Read the model definition and answer for the solid it produces. Units are mm, in the model's axes. A direction names the side the tool comes from. Coordinates: 2 decimals unless noted, no trailing zeros. Write each loop counter-clockwise with the first axis right and the second up, starting at its lowest first coordinate (ties: lowest second). Pieces come first, ordered by that corner, then holes. Notation, with made-up numbers: (-4, 14) - (41, 14) arc R13 ccw to (41, 29) - close; hole circle Ø7 at (-26.75, 47.25). An arc over 180 degrees is marked (long way). Use a Markdown table: item, result.
from build123d import *

# Parameters (mm, degrees)
SKETCH2_W            = 54.6
SKETCH2_H            = 28
SKETCH2_R            = 2.04
SKETCH2_W_2          = 40.6
SKETCH2_H_2          = 20.5
BOSS_EXTRUDE1_DEPTH  = 7.5
SKETCH3_W            = 40.6
SKETCH3_H            = 3.75
BOSS_EXTRUDE2_DEPTH  = 18.4
SKETCH7_W            = 74.600133011
SKETCH7_H            = 74.600133011
BOSS_EXTRUDE4_DEPTH  = 5
CUT_EXTRUDE2_DEPTH   = 5
SKETCH9_R            = 1.55
CUT_EXTRUDE3_DEPTH   = 16
FILLET3_R            = 1
FILLET3_OF_MIRROR4_R = 1
FILLET4_R            = 3


# Read off the part's stored shape, not the designer's step: Mirror5
with BuildPart() as part:
    # Sketch2 → Boss-Extrude1 (new body)
    with BuildSketch(Plane.XY):
        Rectangle(SKETCH2_W, SKETCH2_H)
        with Locations((23.85, 4.9)):
            Circle(SKETCH2_R, mode=Mode.SUBTRACT)
        with Locations(Location((23.85, -4.9, 0), (0, 0, 180))):
            Circle(SKETCH2_R, mode=Mode.SUBTRACT)
        with Locations((-23.85, -4.9)):
            Circle(SKETCH2_R, mode=Mode.SUBTRACT)
        with Locations(Location((-23.85, 4.9, 0), (0, 0, 180))):
            Circle(SKETCH2_R, mode=Mode.SUBTRACT)
        Rectangle(SKETCH2_W_2, SKETCH2_H_2, mode=Mode.SUBTRACT)
    extrude(amount=BOSS_EXTRUDE1_DEPTH)

    # Sketch3 → Boss-Extrude2 (add)
    with BuildSketch(Plane.XY.offset(7.5)):
        with Locations((0, 12.125)):
            Rectangle(SKETCH3_W, SKETCH3_H)
        with Locations((0, -12.125)):
            Rectangle(SKETCH3_W, SKETCH3_H)
    extrude(amount=BOSS_EXTRUDE2_DEPTH)

    # Sketch7 → Boss-Extrude4 (add)
    with BuildSketch(Plane.XY.offset(25.9)):
        with Locations((10.000066505, -7.842e-05)):
            Rectangle(SKETCH7_W, SKETCH7_H)
    extrude(amount=BOSS_EXTRUDE4_DEPTH)

    # Sketch8 → Cut-Extrude2 (cut)
    with BuildSketch(Plane.XY.offset(30.9)):
        Polygon((-27.3, 15.299988086), (-20.542640687, 22.057347399), (-26.906601718, 28.421308429), (-24.078174593, 31.249735554), (-17.714213562, 24.885774524), (-14.885786438, 27.714201648), (-21.249747468, 34.078162679), (-18.421320344, 36.906589804), (-12.057359313, 30.542628773), (-5.3, 37.299988086), (-27.3, 37.299988086), align=None)
    cut_extrude2 = extrude(amount=-CUT_EXTRUDE2_DEPTH, mode=Mode.SUBTRACT)

    # Sketch9 → Cut-Extrude3 (cut)
    with BuildSketch(Plane(origin=(0.757353356, 0.757353356, 0), x_dir=(0, 0, 1), z_dir=(-0.7071067811865474, -0.7071067811865477, 0))):
        with Locations(Location((28.4, 36.122740454, 0), (0, 0, 270))):
            Circle(SKETCH9_R)
    cut_extrude3 = extrude(amount=-CUT_EXTRUDE3_DEPTH, mode=Mode.SUBTRACT)

    # Fillet3
    fillet3_edges = [part.edges().sort_by_distance(p)[0] for p in [
        (-25.492388155, 29.835521992, 30.9),
        (-19.835533906, 35.492376241, 30.9),
        (-19.835533906, 35.492376241, 25.9),
        (-25.492388155, 29.835521992, 25.9),
    ]]
    fillet(fillet3_edges, radius=FILLET3_R)

    # Mirror4: Cut-Extrude2, Cut-Extrude3 across plane
    add(cut_extrude2.mirror(Plane.ZY.offset(-10.000066506)), mode=Mode.SUBTRACT)
    add(cut_extrude3.mirror(Plane.ZY.offset(-10.000066506)), mode=Mode.SUBTRACT)

    # Fillet3 of Mirror4
    fillet3_of_mirror4_edges = [part.edges().sort_by_distance(p)[0] for p in [
        (45.492521167, 29.835521992, 30.9),
        (39.835666917, 35.492376241, 30.9),
        (39.835666917, 35.492376241, 25.9),
        (45.492521167, 29.835521992, 25.9),
    ]]
    fillet(fillet3_of_mirror4_edges, radius=FILLET3_OF_MIRROR4_R)

    # Mirror5
    split(bisect_by=Plane.ZX.offset(-7.842e-05), keep=Keep.TOP)

    # Mirror5 2: part across plane


with BuildPart() as part_1:
    add(part.part)
    add(part.part.mirror(Plane.ZX.offset(-7.842e-05)))

    # Fillet4
    fillet4_edges = [part_1.edges().sort_by_distance(p)[0] for p in [
        (-20.3, 12.125, 7.5),
        (20.3, 12.125, 7.5),
        (0, 14, 25.9),
        (-20.3, 12.125, 25.9),
        (20.3, 12.125, 25.9),
        (-20.3, -12.125156839, 7.5),
        (20.3, -12.125156839, 7.5),
        (-20.3, -12.125156839, 25.9),
        (0, -14.000156839, 25.9),
        (20.3, -12.125156839, 25.9),
        (-27.3, -14.000156839, 3.75),
        (-27.3, 14, 3.75),
        (27.3, 14, 3.75),
        (27.3, -14.000156839, 3.75),
    ]]
    fillet(fillet4_edges, radius=FILLET4_R)


solid = part_1.part
(1) For faces 4 (the cylindrical face through (26.44, 13.1, 3.8)), 5 (the flat face through (42.973, 24.488, 28.435)), 6 (the cylindrical face through (25.8, -5.5, 3.7)), determine the directions among +Z, -Z, +X, -X, +Y, -Y from which every point of the face is accessible in a straight line to the end or side of a thin tool.
Report:
| item | result |
|---|---|
| face 4 | -Z, +X, +Y |
| face 5 | +Z, -Z, +X |
| face 6 | -Z |
(2) The mould has two halves that part along Z. Classify faces 1 (the cylindrical face through (-21.2, 12.15, 8.36)), 2 (the cylindrical face through (0.33, 14.9, 25.04)), 3 (the flat face through (37.316, -30.145, 28.435)): pulls with the +Z half, pulls with the -Z half, needs draft (parallel to the pull), parting line crosses it, or undercut.
Report:
| item | result |
|---|---|
| face 1 | undercut |
| face 2 | pulls with the -Z half |
| face 3 | needs draft |
(3) A cutting plane is placed at A-A, the plane y = 4.9. Write down the section's boundary in (x, z), and give its area (3 significant figures).
Report:
| item | result |
|---|---|
| outline | (-27.3, 0) - (-25.89, 0) - (-25.89, 7.5) - (-27.3, 7.5) - close; (-27.3, 25.9) - (47.3, 25.9) - (47.3, 30.9) - (-27.3, 30.9) - close; (-21.81, 0) - (-20.3, 0) - (-20.3, 7.5) - (-21.81, 7.5) - close; (20.3, 0) - (21.81, 0) - (21.81, 7.5) - (20.3, 7.5) - close; (25.89, 0) - (27.3, 0) - (27.3, 7.5) - (25.89, 7.5) - close |
| area | 417 mm² |
(4) A cutting plane is placed at D-D, the plane y = -8.5. Write down the section's boundary in (x, z), and give its area (3 significant figures).
Report:
| item | result |
|---|---|
| outline | (-27.3, 0) - (-20.3, 0) - (-20.3, 7.5) - (-27.3, 7.5) - close; (-27.3, 25.9) - (47.3, 25.9) - (47.3, 30.9) - (-27.3, 30.9) - close; (20.3, 0) - (27.3, 0) - (27.3, 7.5) - (20.3, 7.5) - close |
| area | 478 mm² |
(5) Each of these flat-tipped pins is pushed along its axis until it touches: P1, Ø2, axis at y = 1.5, z = 4, coming from the +X side; P2, Ø18.5, axis at x = -11, z = 11.5, coming from the -Y side; P3, Ø13, axis at x = 1, z = 13, coming from the +Y side. Where does it stop, or does it pass through?
Report:
| item | result |
|---|---|
| P1 | stops at x = 27.3 |
| P2 | stops at y = -14 |
| P3 | stops at y = 14 |
(6) A cutting plane is placed at B-B, the plane z = 13.5. Write down the section's boundary in (x, y), and give its area (4 significant figures).
Report:
| item | result |
|---|---|
| outline | (-20.3, -14) - (20.3, -14) - (20.3, -10.25) - (-20.3, -10.25) - close; (-20.3, 10.25) - (20.3, 10.25) - (20.3, 14) - (-20.3, 14) - close |
| area | 304.5 mm² |
(7) A cutting plane is placed at C-C, the plane x = 11.5. Write down the section's boundary in (y, z), and give its area (3 significant figures).
Report:
| item | result |
|---|---|
| outline | (-37.3, 25.9) - (-17, 25.9) arc R3 cw to (-14, 22.9) - (-14, 0) - (-10.25, 0) - (-10.25, 25.9) - (10.25, 25.9) - (10.25, 0) - (14, 0) - (14, 22.9) arc R3 cw to (17, 25.9) - (37.3, 25.9) - (37.3, 30.9) - (-37.3, 30.9) - close |
| area | 571 mm² |
(8) Straight lines are drawn through the part: L1, parallel to X at y = 4, z = 5; L2, parallel to X at y = 0.5, z = 4; L3, parallel to Y at x = -4, z = 10. For each, find the intervals that lie inside material, in ascending order.
Report:
| item | result |
|---|---|
| L1 | x = -27.3 to -25.68, -22.02 to -20.3, 20.3 to 22.02, 25.68 to 27.3 |
| L2 | x = -27.3 to -20.3, 20.3 to 27.3 |
| L3 | y = -14 to -10.25, 10.25 to 14 |
